Geometry check sheet. Reference: the model listing, model coordinates, mm. Face numbers are marked on the shaded views. A direction names the side the tool comes from. Round coordinates to 2 decimals unless told otherwise and drop trailing zeros. Loops run counter-clockwise (first coordinate to the right, second up) from the corner with the lowest first, then second, coordinate; pieces in that order, holes last. Notation, with made-up numbers: (-26.5, -26.75) - (17.5, -26.75) arc R33 ccw to (17.5, 3.25) - close; hole circle Ø8 at (58, 26). An arc over 180 degrees is marked (long way). Write item = value, one per line.
```python
from build123d import *

# Parameters (mm, degrees)
SKETCH1_R                      = 53
BOSS_EXTRUDE1_DEPTH            = 50
F_10_0_10_DIAMETER_HOLE2_D     = 10
F_10_0_10_DIAMETER_HOLE2_DEPTH = 17.5
F_10_0_10_DIAMETER_HOLE2_TIP   = 3.004303095
M4_TAPPED_HOLE1_REACH          = 130.627
M4_TAPPED_HOLE1_BORE_R         = 1.65
CIRPATTERN1_COUNT              = 3
CIRPATTERN1_ANGLE              = 180
SKETCH11_R                     = 30
CUT_EXTRUDE2_DEPTH             = 45
SKETCH12_W                     = 4.826
SKETCH12_H                     = 2.76515
SKETCH12_W_2                   = 7.2136
SKETCH12_H_2                   = 4.27264
SKETCH14_W                     = 2.667
SKETCH14_H                     = 4.572
CIRPATTERN2_COUNT              = 4


with BuildPart() as part:
    # Sketch1 → Boss-Extrude1 (new body)
    with BuildSketch(Plane.XY):
        Circle(SKETCH1_R)
    extrude(amount=BOSS_EXTRUDE1_DEPTH)

    # Ø10.0 (10) Diameter Hole2
    with Locations(Plane.XY.offset(50)):
        with Locations((-37, 0), (37, 0), (0, -40)):
            Hole(F_10_0_10_DIAMETER_HOLE2_D / 2, depth=F_10_0_10_DIAMETER_HOLE2_DEPTH)
            with Locations((0, 0, -(F_10_0_10_DIAMETER_HOLE2_DEPTH + F_10_0_10_DIAMETER_HOLE2_TIP / 2))):  # 118° drill point
                Cone(0, F_10_0_10_DIAMETER_HOLE2_D / 2, F_10_0_10_DIAMETER_HOLE2_TIP, mode=Mode.SUBTRACT)

    # M4 Tapped Hole1 bore → M4 Tapped Hole1 (cut, up to next)
    with BuildSketch(Plane.ZY.offset(53), mode=Mode.PRIVATE) as m4_tapped_hole1_sk1:
        with Locations((44, 0)):
            Circle(M4_TAPPED_HOLE1_BORE_R)
    m4_tapped_hole1_tool1 = extrude(m4_tapped_hole1_sk1.sketch, amount=-M4_TAPPED_HOLE1_REACH, mode=Mode.PRIVATE) & part.part
    m4_tapped_hole1 = m4_tapped_hole1_tool1.solids().sort_by_distance((-53, 0, 44))[0]
    add(m4_tapped_hole1, mode=Mode.SUBTRACT)

    # CirPattern1: M4 Tapped Hole1 ×3 about axis
    cirpattern1_axis = Axis((0, 0, 50), (0, 0, 1))
    for i in range(1, CIRPATTERN1_COUNT):
        add(m4_tapped_hole1.rotate(cirpattern1_axis, i * CIRPATTERN1_ANGLE / (CIRPATTERN1_COUNT - 1)), mode=Mode.SUBTRACT)

    # Sketch11 → Cut-Extrude2 (cut)
    with BuildSketch(Plane.XY.offset(50)):
        Circle(SKETCH11_R)
    extrude(amount=-CUT_EXTRUDE2_DEPTH, mode=Mode.SUBTRACT)

    # Sketch12 → Cut-Revolve1 (revolve, cut)
    with BuildSketch(Plane(origin=(0, 0, 0), x_dir=(0, 0, -1), z_dir=(1, 0, 0)), mode=Mode.PRIVATE) as cut_revolve1_sk:
        with Locations((-12.413, 51.617425)):
            Rectangle(SKETCH12_W, SKETCH12_H)
        with Locations((-23.4328, 50.86368)):
            Rectangle(SKETCH12_W_2, SKETCH12_H_2)
    revolve(cut_revolve1_sk.sketch.rotate(Axis((0, 0, 0), (0, 0, 1)), 90), axis=Axis((0, 0, 0), (0, 0, 1)), mode=Mode.SUBTRACT)

    # Sketch14 → Cut-Revolve2 (revolve, cut)
    with BuildSketch(Plane(origin=(0, 0, 0), x_dir=(0, 0, -1), z_dir=(1, 0, 0)), mode=Mode.PRIVATE) as cut_revolve2_sk:
        with Locations((-1.3335, 24.8666)):
            Rectangle(SKETCH14_W, SKETCH14_H)
    revolve(cut_revolve2_sk.sketch.rotate(Axis((0, 0, 0), (0, 0, -1)), 270), axis=Axis((0, 0, 0), (0, 0, -1)), mode=Mode.SUBTRACT)

    # Sketch17 → M5 Tapped Hole1 (revolve, cut)
    with BuildSketch(Plane(origin=(-28.284271247, 28.284271247, 0), x_dir=(0, 1, 0), z_dir=(1, 0, 0))):
        Polygon((0, 0), (0, 15.2618073), (2.1, 14), (2.1, 0), align=None)
    m5_tapped_hole1 = revolve(axis=Axis((-28.284271247, 28.284271247, -6.35), (0, 0, 1)), mode=Mode.SUBTRACT)

    # CirPattern2: M5 Tapped Hole1 ×4 about axis
    cirpattern2_axis = Axis((0, 0, 0), (0, 0, 1))
    for i in range(1, CIRPATTERN2_COUNT):
        add(m5_tapped_hole1.rotate(cirpattern2_axis, i * 360 / CIRPATTERN2_COUNT), mode=Mode.SUBTRACT)


solid = part.part
```
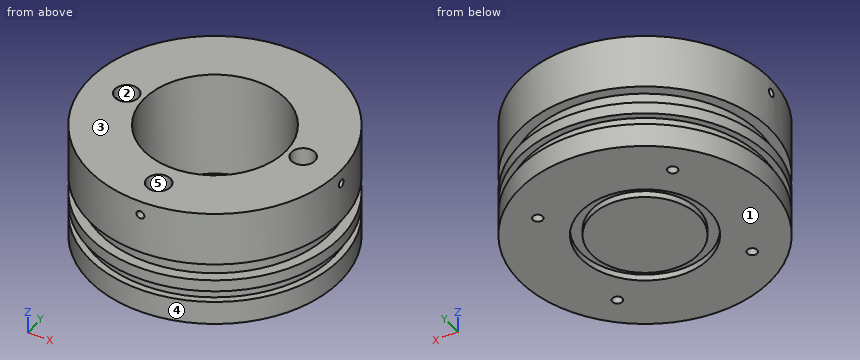
(1) Section check B-B (z = 38.5). Enter the section's corners in (x, y).
Answers follow:
outline = circle Ø106 at (0, 0); hole circle Ø10 at (-37, 0); hole circle Ø60 at (0, 0); hole circle Ø10 at (0, -40); hole circle Ø10 at (37, 0)
(2) Section check C-C (y = 45.5). Enter the section's corners in (x, z).
Answers follow:
outline = (-27.18, 0) - (27.18, 0) - (27.18, 10) - (21.29, 10) - (21.29, 14.83) - (27.18, 14.83) - (27.18, 19.83) - (17.44, 19.83) - (17.44, 27.04) - (27.18, 27.04) - (27.18, 50) - (-27.18, 50) - (-27.18, 27.04) - (-17.44, 27.04) - (-17.44, 19.83) - (-27.18, 19.83) - (-27.18, 14.83) - (-21.29, 14.83) - (-21.29, 10) - (-27.18, 10) - close
(3) Set-up check for the marked faces 1 and 2: record each of +Z, -Z, +X, -X, +Y, -Y from which the full face is reachable in a straight line by a thin tool's end or side.
Answers follow:
face_1 = -Z, +X, -X, +Y, -Y
face_2 = +Z
(4) Section check A-A (x = 44.5). Enter the section's corners in (y, z).
Answers follow:
outline = (-28.79, 0) - (28.79, 0) - (28.79, 10) - (23.31, 10) - (23.31, 14.83) - (28.79, 14.83) - (28.79, 19.83) - (19.85, 19.83) - (19.85, 27.04) - (28.79, 27.04) - (28.79, 50) - (-28.79, 50) - (-28.79, 27.04) - (-19.85, 27.04) - (-19.85, 19.83) - (-28.79, 19.83) - (-28.79, 14.83) - (-23.31, 14.83) - (-23.31, 10) - (-28.79, 10) - close; hole circle Ø3.3 at (0, 44)
(5) Mould release check, pull along X, two halves, no side actions. Record for the marked faces 3, 4 and 5: pulls with the +X half, pulls with the -X half, needs draft (parallel to the pull), parting line crosses it, or undercut.
Answers follow:
face_3 = needs draft
face_4 = parting line crosses it
face_5 = undercut
(6) Gauge pin test, flat ends, axial feed: pin 1 (6 mm diameter, centred on y = -29, z = 19.5, fed in from -X); pin 2 (8 mm diameter, centred on x = 18, z = 43, fed in from -Y); pin 3 (10 mm diameter, centred on y = 20, z = 28.5, fed in from +X). Record the tip position at first contact, or that the pin passes through.
Answers follow:
pin_1 = -46.18
pin_2 = -51.12
pin_3 = 50.83
(7) Scan lines: L1, parallel to Z at x = 21, y = 48; L2, parallel to Y at x = 0, z = 1.9; L3, parallel to Y at x = 0, z = 44. Record each from-to range of solid material in increasing order. Write a range as [from, to].
Answers follow:
L1 = [0, 10], [14.83, 19.83], [27.04, 50]
L2 = [-53, -27.15], [-22.58, 22.58], [27.15, 53]
L3 = [-35, -30], [30, 53]
